Input: part model. Units: mm. Frame: model coordinates. A direction names the side the tool comes from. Round coordinates to 2 decimals unless told otherwise and drop trailing zeros. Loops run counter-clockwise (first coordinate to the right, second up) from the corner with the lowest first, then second, coordinate; pieces in that order, holes last. Notation, with made-up numbers: (52, 49) - (72, 49) arc R20 ccw to (72, 78) - close; hole circle Ø6 at (-1.75, 18.5). An arc over 180 degrees is marked (long way). One line per question, with ' | ' between items. Start each with the question number.
Autodesk Fusion 360 part; units mm, degrees
sketch "Sketch1" plane through (0, 0, 0) normal (0, 0, 1) x (1, 0, 0)
  circle A0 centre (0, 0) radius 4
  circle A1 centre (-0.5, 0) radius 2.5
  line L0 (-2.5, 1.5) -> (-2.5, -1.5)
  circle A2 centre (-2, 1.5) radius 0.5
  line L1 (-2.8087, 1.6679) -> (-0.6979, 2.676)
  line L2 (-0.5, 0) -> (0, 0)
  line L3 (-2.8087, -1.6679) -> (-0.6979, -2.676)
  circle A3 centre (-2, -1.5) radius 0.5
  dimension "d1" = 8
  dimension "d2" = 5
  dimension "d3" = 0.5
  dimension "d4" = 2
  dimension "d13" = 1
extrude "Extrude3" add sketch "Sketch1" along normal blind 2.5 contours A0 | A1 L0
(1) Pin query (flat end, axial travel): P1, Ø1.5, axis at y = -1, z = 1, coming from the -X side; P2, Ø3, axis at x = -0.5, y = 0, coming from the +Z side; P3, Ø1, axis at x = -3, z = 1.5, coming from the -Y side; P4, Ø1.2, axis at y = 0.5, z = 1, coming from the +X side. Return the tip coordinate at first contact, or that it passes through.
(2) Line query: line 1 along Y through (x, z) = (-0.5, 1.1); line 2 along Y through (x, z) = (-1.25, 0.15); line 3 along X through (y, z) = (-0.25, 1.65). Output: solid intervals per line, ascending. Write a range as from..to.
(3) Section A-A, the plane y = 0. Output: boundary loops of the cut face in (x, z).
(4) Section B-B, the plane x = 0. Output: boundary loops of the cut face in (y, z).
(5) Pull-direction query (X, two-part tool) for faces 3 (the face through (-0.867, 3.905, 1.232)), 4 (the face through (2, 0, 1)), 5 (the face through (2, -2, 2.5)); classes: released by +X, released by -X, zero draft, split by the parting line, or undercut.
(6) Section C-C, the plane z = 0.5. Output: boundary loops of the cut face in (x, y).
(7) Reachability of faces 1 (the face through (-2.5, 0, 1)), 2 (the face through (2, -2, 0)) from +Z, -Z, +X, -X, +Y, -Y: full face, straight path, thin tool, end or side. Return the list, or none.
Derived:
1) P1: stops at x = -3.99 | P2: passes through | P3: stops at y = -3.12 | P4: stops at x = 4
2) line 1: y = -3.97..-2.5, 2.5..3.97 | line 2: y = -3.8..-2.38, 2.38..3.8 | line 3: x = -3.99..-2.5, 1.99..3.99
3) outline: (-4, 0) - (-2.5, 0) - (-2.5, 2.5) - (-4, 2.5) - close; (2, 0) - (4, 0) - (4, 2.5) - (2, 2.5) - close
4) outline: (-4, 0) - (-2.45, 0) - (-2.45, 2.5) - (-4, 2.5) - close; (2.45, 0) - (4, 0) - (4, 2.5) - (2.45, 2.5) - close
5) face 3: split by the parting line | face 4: undercut | face 5: zero draft
6) outline: circle Ø8 at (0, 0); hole (-2.5, -1.5) arc R0.5 ccw to (-2.22, -1.95) - (-1.58, -2.26) arc R2.5 ccw (long way) to (-1.58, 2.26) - (-2.22, 1.95) arc R0.5 ccw to (-2.5, 1.5) - close
7) face 1: +Z, -Z | face 2: -Z, +X, -X, +Y, -Y
